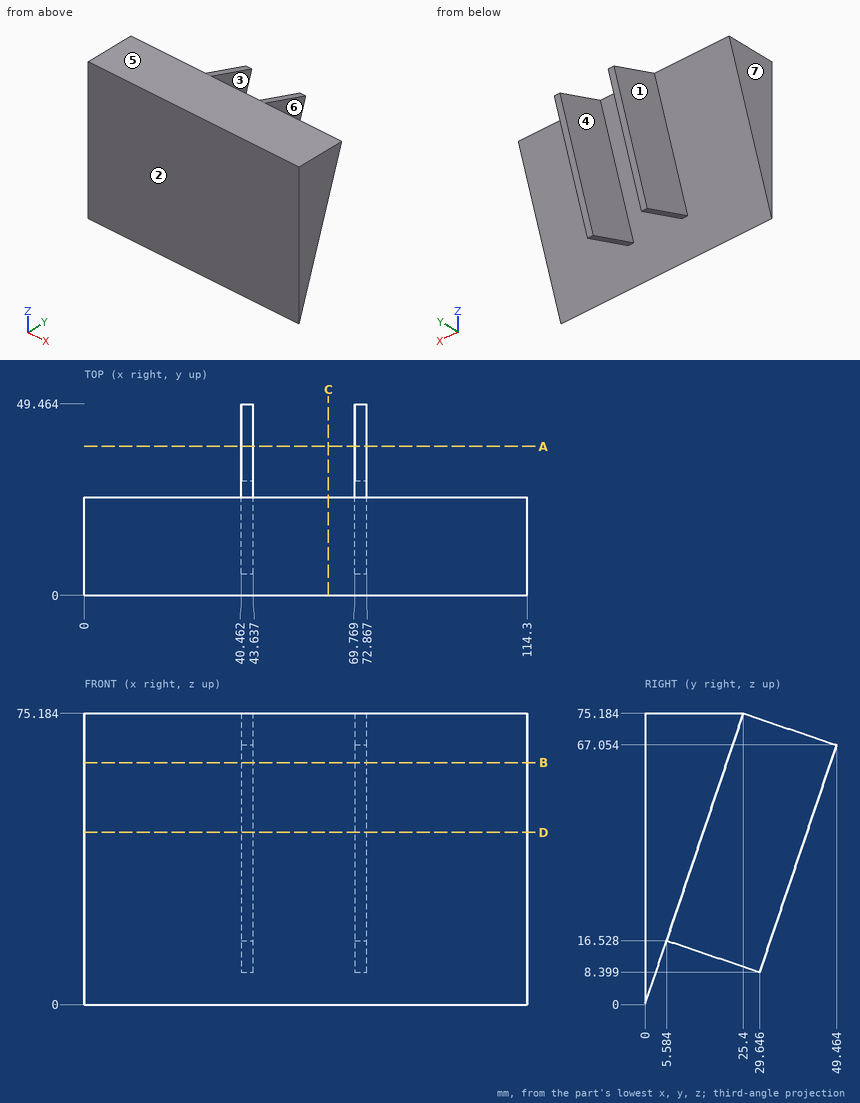
Drawing for the job (mm, zero at the part's lowest x, y, z). A direction names the side the tool comes from. Round coordinates to 2 decimals unless told otherwise and drop trailing zeros. Loops run counter-clockwise (first coordinate to the right, second up) from the corner with the lowest first, then second, coordinate; pieces in that order, holes last. Notation, with made-up numbers: (85, 3) -> (122, 3) arc R18 ccw to (122, 28) -> close; hole circle Ø1 at (-22, 55.5). An arc over 180 degrees is marked (long way). Answer in a Markdown table with one row per item.
Item 1: Pin check, flat tips, straight feed: pin 1 (3 mm diameter, centred on y = 29.5, z = 38, fed in from +X); pin 2 (5 mm diameter, centred on y = 32, z = 16, fed in from -X). Stop position of each tip, or through.
Answers below:
| item | result |
|---|---|
| pin 1 | stops at x = 72.87 |
| pin 2 | stops at x = 40.46 |
Item 2: Saw through at D-D (z = 44.5). Write the cut outline in (x, y).
Answers below:
| item | result |
|---|---|
| outline | (0, 0) -> (114.3, 0) -> (114.3, 15.03) -> (72.87, 15.03) -> (72.87, 41.84) -> (69.77, 41.84) -> (69.77, 15.03) -> (43.64, 15.03) -> (43.64, 41.84) -> (40.46, 41.84) -> (40.46, 15.03) -> (0, 15.03) -> close |
Item 3: Drill centre lines: L1, parallel to X at y = 13, z = 36.5; L2, parallel to Y at x = 102, z = 53 (1 decimal); L3, parallel to Y at x = 102, z = 34.5 (1 decimal). Where is each one in solid material? Low to high. Write a range as [from, to].
Answers below:
| item | result |
|---|---|
| L1 | x = [40.46, 43.64], [69.77, 72.87] |
| L2 | y = [0, 17.9] |
| L3 | y = [0, 11.7] |
Item 4: Which spindle directions (+Z, -Z, +X, -X, +Y, -Y) get a long thin tool onto all of the face, cutting with end or side? Do the marked faces 1, 2 and 3. Say none if no direction does.
Answers below:
| item | result |
|---|---|
| face 1 | -Z, -X, +Y |
| face 2 | +Z, -Z, +X, -X, -Y |
| face 3 | -Z, +Y |
Item 5: Saw through at A-A (y = 38.5). Write the cut outline in (x, z) (1 decimal).
Answers below:
| item | result |
|---|---|
| outline | (40.5, 34.6) -> (43.6, 34.6) -> (43.6, 70.8) -> (40.5, 70.8) -> close; (69.8, 34.6) -> (72.9, 34.6) -> (72.9, 70.8) -> (69.8, 70.8) -> close |
Item 6: Saw through at B-B (z = 62.5). Write the cut outline in (x, y) (1 decimal).
Answers below:
| item | result |
|---|---|
| outline | (0, 0) -> (114.3, 0) -> (114.3, 21.1) -> (72.9, 21.1) -> (72.9, 47.9) -> (69.8, 47.9) -> (69.8, 21.1) -> (43.6, 21.1) -> (43.6, 47.9) -> (40.5, 47.9) -> (40.5, 21.1) -> (0, 21.1) -> close |
Item 7: Mould opens along X. For the marked faces 4, 5, 6 and 7 say: +X half, -X half, draft (parallel to the pull), parting line (faces both ways), or undercut.
Answers below:
| item | result |
|---|---|
| face 4 | undercut |
| face 5 | draft |
| face 6 | +X half |
| face 7 | -X half |
Item 8: Saw through at C-C (x = 63). Write the cut outline in (y, z), and give its area (3 significant figures).
Answers below:
| item | result |
|---|---|
| outline | (0, 0) -> (25.4, 75.18) -> (0, 75.18) -> close |
| area | 955 mm² |
